from build123d import *

# Parameters (mm, degrees)
SKETCH1_W           = 100
SKETCH1_H           = 100
BOSS_EXTRUDE1_DEPTH = 150
SKETCH2_R           = 50
SKETCH2_R_2         = 25
BOSS_EXTRUDE2_DEPTH = 100
SKETCH3_W           = 100
SKETCH3_H           = 50
CUT_EXTRUDE1_DEPTH  = 100
SKETCH4_R           = 25
CUT_EXTRUDE2_DEPTH  = 188.082869339
FILLET1_R           = 50
FILLET2_R           = 10


with BuildPart() as part:
    # Sketch1 → Boss-Extrude1 (new body)
    with BuildSketch(Plane(origin=(0, 0, 0), x_dir=(1, 0, 0), z_dir=(0, 1, 0))):
        Rectangle(SKETCH1_W, SKETCH1_H)
    extrude(amount=BOSS_EXTRUDE1_DEPTH)

    # Sketch2 → Boss-Extrude2 (add)
    with BuildSketch(Plane.XZ):
        with Locations(Location((0, 0, 0), (0, 0, 270))):
            Circle(SKETCH2_R)
        with Locations(Location((0, 0, 0), (0, 0, 270))):
            Circle(SKETCH2_R_2, mode=Mode.SUBTRACT)
    extrude(amount=BOSS_EXTRUDE2_DEPTH)

    # Sketch3 → Cut-Extrude1 (cut)
    with BuildSketch(Plane(origin=(0, 150, 0), x_dir=(1, 0, 0), z_dir=(0, 1, 0))):
        Rectangle(SKETCH3_W, SKETCH3_H)
    extrude(amount=-CUT_EXTRUDE1_DEPTH, mode=Mode.SUBTRACT)

    # Sketch4 → Cut-Extrude2 (cut, through all)
    with BuildSketch(Plane.XY.offset(50)):
        with Locations((0, 100)):
            Circle(SKETCH4_R)
    extrude(amount=-CUT_EXTRUDE2_DEPTH, mode=Mode.SUBTRACT)

    # Fillet1
    fillet1_edges = [part.edges().sort_by_distance(p)[0] for p in [
        (50, 150, 37.5),
        (50, 150, -37.5),
        (-50, 150, -37.5),
        (-50, 150, 37.5),
    ]]
    fillet(fillet1_edges, radius=FILLET1_R - 0.0001)  # a hair under: the kernel refuses the full size

    # Fillet2
    fillet2_edges = [part.edges().sort_by_distance(p)[0] for p in [
        (50, 50.00005, 50),
        (50, 50.00005, -50),
        (-50, 50.00005, 50),
        (-35.355368349, 135.355368349, 50),
        (35.355368349, 135.355368349, 50),
        (-50, 50.00005, -50),
        (-35.355368349, 135.355368349, -50),
        (35.355368349, 135.355368349, -50),
    ]]
    fillet(fillet2_edges, radius=FILLET2_R)


solid = part.part
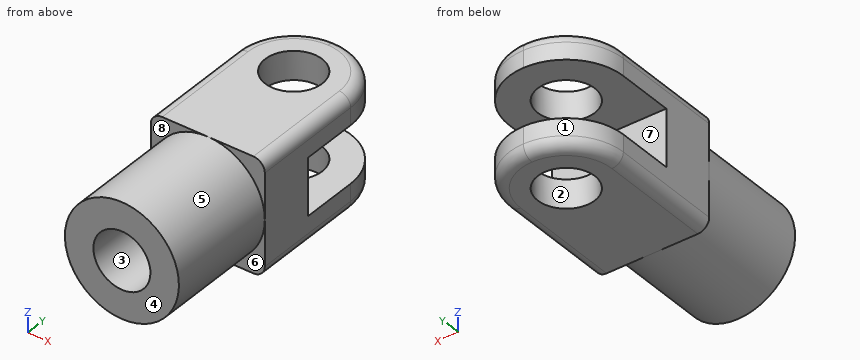
Build history of the part. All positions in model axes, mm. Face numbers are marked on the shaded views. A direction names the side the tool comes from. Round coordinates to 2 decimals unless told otherwise and drop trailing zeros. Loops run counter-clockwise (first coordinate to the right, second up) from the corner with the lowest first, then second, coordinate; pieces in that order, holes last. Notation, with made-up numbers: (-1.5, 79) -> (6.5, 79) arc R20 ccw to (6.5, 94) -> close; hole circle Ø10 at (10, 6.25). An arc over 180 degrees is marked (long way). Use CSV: the item, a comma, the result in double quotes. Start each with the question number.
Q1. Saw through at D-D on z = 5.5. Give the cut face in (x, y), and give its area (3 significant figures).
Q2. Drill centre lines: L1, parallel to X at y = -27.5, z = 0; L2, parallel to Y at x = 0, z = -35; L3, parallel to Y at x = -41, z = -5. Where is each one in solid material? Low to high.
Q3. Saw through at C-C on x = -10. Count the separate pieces of the cut face and the enclosed holes in it, and give its area (3 significant figures).
Q4. Flat gauge pins, fed straight in: pin 1 Ø25 at (x, z) = (21.5, 8.5) entering from +Y; pin 2 Ø1.5 at (x, z) = (-2.5, 21) entering from -Y; pin 3 Ø6 at (x, y) = (-17.5, -27.5) entering from -Z. Where does each tip first touch, or does it go through?
Q5. Saw through at B-B on z = 17.5. Give the cut face in (x, y), and give its area (3 significant figures).
Q6. Which spindle directions (+Z, -Z, +X, -X, +Y, -Y) get a long thin tool onto all of the face, cutting with end or side? Do the marked faces 5, 6, 7 and 8. Say none if no direction does.
Q7. Mould opens along X. For the marked faces 1, 2, 3 and 4 say: +X half, -X half, draft (parallel to the pull), parting line (faces both ways), or undercut.
Solutions:
1,outline,"(-50, 0) -> (-49.7, 0) -> (-49.7, -100) -> (-24.39, -100) -> (-24.39, 0) -> (24.39, 0) -> (24.39, -100) -> (49.7, -100) -> (49.7, 0) -> (50, 0) -> (50, 50) -> (-50, 50) -> close"
1,area,"10,100 mm^2"
2,L1,"x = -50 to -25, 25 to 50"
2,L2,"y = -100 to 75, 125 to 150"
2,L3,"y = -100 to 50"
3,separate pieces,"3"
3,enclosed holes,"0"
3,area,"12,800 mm^2"
4,pin 1,"stops at y = 50"
4,pin 2,"stops at y = 0"
4,pin 3,"stops at z = -47.85"
5,outline,"(-50, 0) -> (-46.84, 0) -> (-46.84, -100) -> (-17.85, -100) -> (-17.85, 0) -> (17.85, 0) -> (17.85, -100) -> (46.84, -100) -> (46.84, 0) -> (50, 0) -> (50, 50) -> (-50, 50) -> close"
5,area,"10,800 mm^2"
6,face 5,"-Y"
6,face 6,"-Z, +X, -Y"
6,face 7,"+X, -X, +Y"
6,face 8,"+Z, -X, -Y"
7,face 1,"-X half"
7,face 2,"undercut"
7,face 3,"undercut"
7,face 4,"draft"
